Work out the finished part from the listing and answer in its coordinate system (mm). Face numbers are marked on the shaded views. A direction names the side the tool comes from. Round coordinates to 2 decimals unless told otherwise and drop trailing zeros. Write each loop counter-clockwise with the first axis right and the second up, starting at its lowest first coordinate (ties: lowest second). Pieces come first, ordered by that corner, then holes.
1. Find section D-D (z = 31). Write down the section's boundary in (x, y).
2. Find section A-A (y = 0). Write down the section's boundary in (x, z), and give its area (3 significant figures).
3. A tool of negligible diameter and unlimited length cuts with its end or side. For the marked faces 4, 5 and 6, from which of +Z, -Z, +X, -X, +Y, -Y can it reach the whole face along a straight path? Write none if from no direction.
4. Determine the mould class of the marked faces 1, 2 and 3 for opening direction Y: pulls with the +Y half, pulls with the -Y half, needs draft (parallel to the pull), parting line crosses it, or undercut.
5. Straight lines are drawn through the part: probe 1 along Y at (x, z) = (9, 19.05); probe 2 along Y at (x, z) = (0, 21.75); probe 3 along Z at (x, y) = (7.5, 0). For each, find the intervals that lie inside material, in ascending order.
6. Find section B-B (x = 0). Write down the section's boundary in (y, z), and give its area (3 significant figures).
7. Find section C-C (x = 11). Write down the section's boundary in (y, z), and give its area (3 significant figures).
```python
from build123d import *

# Parameters (mm, degrees)
SKETCH2_W                          = 25.4
SKETCH2_H                          = 25.4
BOSS_EXTRUDE1_DEPTH                = 38.1
F_7_16_20_TAPPED_HOLE2_D           = 9.92124
F_7_16_20_TAPPED_HOLE2_DEPTH       = 12.7
F_7_16_20_TAPPED_HOLE2_CSINK_D     = 12.3825
F_7_16_20_TAPPED_HOLE2_CSINK_ANGLE = 90
F_7_16_20_TAPPED_HOLE2_TIP         = 2.980641204


with BuildPart() as part:
    # Sketch2 → Boss-Extrude1 (new body)
    with BuildSketch(Plane.XY):
        Rectangle(SKETCH2_W, SKETCH2_H)
    extrude(amount=BOSS_EXTRUDE1_DEPTH)

    # Sketch6 → 1/4 NPT Tapped Hole1 (revolve, cut)
    with BuildSketch(Plane(origin=(0, 0, 38.1), x_dir=(0, -1, 0), z_dir=(1, 0, 0))):
        Polygon((0, 0), (0, 38.1), (5.5626, 38.1), (5.5626, 10.02), (5.950661746, 10.02), (6.2436883, 0.2333117), (6.477, 0), align=None)
    revolve(axis=Axis((0, 0, 44.45), (0, 0, -1)), mode=Mode.SUBTRACT)

    # Sketch8 → 1/4 NPT Tapped Hole2 (revolve, cut)
    with BuildSketch(Plane.YZ):
        Polygon((0, 0), (0, 38.1), (5.5626, 38.1), (5.5626, 10.02), (5.950661746, 10.02), (6.2436883, 0.2333117), (6.477, 0), align=None)
    revolve(axis=Axis((0, 0, -6.35), (0, 0, 1)), mode=Mode.SUBTRACT)

    # 7/16-20 Tapped Hole2
    with Locations(Plane(origin=(12.7, 0, 0), x_dir=(0, 0, -1), z_dir=(1, 0, 0))):
        with Locations((-19.05, 0)):
            CounterSinkHole(F_7_16_20_TAPPED_HOLE2_D / 2, F_7_16_20_TAPPED_HOLE2_CSINK_D / 2, depth=F_7_16_20_TAPPED_HOLE2_DEPTH, counter_sink_angle=F_7_16_20_TAPPED_HOLE2_CSINK_ANGLE)
            with Locations((0, 0, -(F_7_16_20_TAPPED_HOLE2_DEPTH + F_7_16_20_TAPPED_HOLE2_TIP / 2))):  # 118° drill point
                Cone(0, F_7_16_20_TAPPED_HOLE2_D / 2, F_7_16_20_TAPPED_HOLE2_TIP, mode=Mode.SUBTRACT)


solid = part.part
```
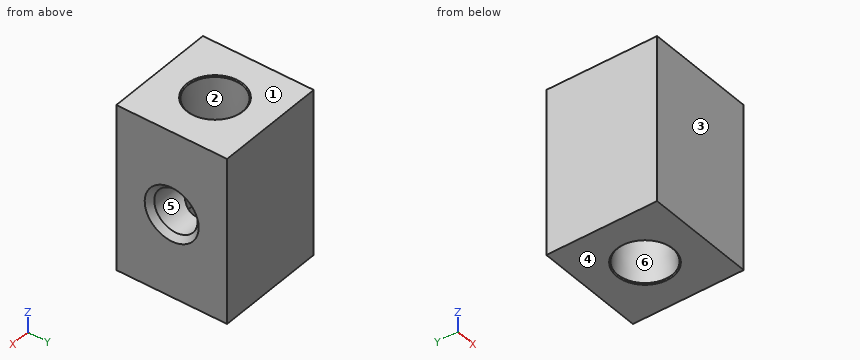
Worked answers:
1. outline: (-12.7, -12.7) - (12.7, -12.7) - (12.7, 12.7) - (-12.7, 12.7) - close; hole circle Ø12.08 at (0, 0)
2. outline: (-12.7, 0) - (-6.48, 0) - (-6.24, 0.23) - (-5.95, 10.02) - (-5.56, 10.02) - (-5.56, 28.08) - (-5.95, 28.08) - (-6.24, 37.87) - (-6.48, 38.1) - (-12.7, 38.1) - close; (5.56, 10.02) - (5.95, 10.02) - (6.24, 0.23) - (6.48, 0) - (12.7, 0) - (12.7, 12.86) - (11.47, 14.09) - (5.56, 14.09) - close; (5.56, 24.01) - (11.47, 24.01) - (12.7, 25.24) - (12.7, 38.1) - (6.48, 38.1) - (6.24, 37.87) - (5.95, 28.08) - (5.56, 28.08) - close
2. area: 450 mm2
3. face 4: -Z, +X, -X, +Y, -Y
3. face 5: +X
3. face 6: -Z
4. face 1: needs draft
4. face 2: undercut
4. face 3: pulls with the -Y half
5. probe 1: y = -12.7 to -4.96, 4.96 to 12.7
5. probe 2: y = -12.7 to -5.56, 5.56 to 12.7
5. probe 3: z = 0 to 14.09, 24.01 to 38.1
6. outline: (-12.7, 0) - (-6.48, 0) - (-6.24, 0.23) - (-5.95, 10.02) - (-5.56, 10.02) - (-5.56, 28.08) - (-5.95, 28.08) - (-6.24, 37.87) - (-6.48, 38.1) - (-12.7, 38.1) - close; (5.56, 10.02) - (5.95, 10.02) - (6.24, 0.23) - (6.48, 0) - (12.7, 0) - (12.7, 38.1) - (6.48, 38.1) - (6.24, 37.87) - (5.95, 28.08) - (5.56, 28.08) - close
6. area: 522 mm2
7. outline: (-12.7, 0) - (12.7, 0) - (12.7, 38.1) - (-12.7, 38.1) - close; hole circle Ø9.92 at (0, 19.05)
7. area: 890 mm2
